Part model, mm, in its own coordinate system. Face numbers are marked on the shaded views. A direction names the side the tool comes from. Give positions to 0.01 mm unless a question says otherwise; leave off trailing zeros. Write each loop counter-clockwise with the first axis right and the second up, starting at its lowest first coordinate (ties: lowest second). Pieces come first, ordered by that corner, then holes. Notation, with made-up numbers: M -19.75,10 L 15.25,10 A18 ccw 15.25,22 Z; hole C -10.75,62.5 d11. An arc over 180 degrees is marked long. Use a Markdown table: item, result.
```python
from build123d import *

# Parameters (mm, degrees)
SKETCH1_W               = 139.999999908
SKETCH1_H               = 52.6999962
BOSS_EXTRUDE1_DEPTH     = 33.02
CUT_EXTRUDE1_DEPTH      = 154.191416123
CUT_EXTRUDE1_DEPTH_BACK = 154.191416123
CUT_EXTRUDE2_DEPTH      = 26
CUT_EXTRUDE3_START      = -26
CUT_EXTRUDE3_DEPTH      = 26
CUT_EXTRUDE4_DEPTH      = 154.191416123
CUT_EXTRUDE4_DEPTH_BACK = 154.191416123
SKETCH6_W               = 26
SKETCH6_H               = 36
CUT_EXTRUDE5_DEPTH      = 154.191416123
CUT_EXTRUDE5_DEPTH_BACK = 154.191416123
SKETCH7_R               = 1.500000048
SKETCH7_R_2             = 1.5


with BuildPart() as part:
    # Sketch1 → Boss-Extrude1 (new body)
    with BuildSketch(Plane.XY):
        with Locations((69.999999954, 26.3499981)):
            Rectangle(SKETCH1_W, SKETCH1_H)
    extrude(amount=BOSS_EXTRUDE1_DEPTH)

    # Sketch2 → Cut-Extrude1 (cut, two sides: drawn at the far end of the back side and taken through both)
    with BuildSketch(Plane.ZY.offset(-CUT_EXTRUDE1_DEPTH_BACK)):
        with BuildLine():
            Line((33.02, 44.3499981), (33.02, 8.3499981))
            ThreePointArc((33.02, 8.3499981), (15.02, 26.3499981), (33.02, 44.3499981))
        make_face()
    extrude(amount=CUT_EXTRUDE1_DEPTH + CUT_EXTRUDE1_DEPTH_BACK, mode=Mode.SUBTRACT)

    # Sketch3 → Cut-Extrude2 (cut)
    with BuildSketch(Plane.ZY):
        with BuildLine():
            Line((33.02, 46.3499981), (33.02, 6.3499981))
            ThreePointArc((33.02, 6.3499981), (13.02, 26.3499981), (33.02, 46.3499981))
        make_face()
    extrude(amount=-CUT_EXTRUDE2_DEPTH, mode=Mode.SUBTRACT)

    # Sketch5 → Cut-Extrude3 (cut)
    with BuildSketch(Plane(origin=(139.999999908, 0, 0), x_dir=(0, 0, -1), z_dir=(1, 0, 0)).offset(CUT_EXTRUDE3_START)):
        with BuildLine():
            Line((-33.02, 46.3499981), (-33.02, 6.3499981))
            ThreePointArc((-33.02, 6.3499981), (-13.02, 26.3499981), (-33.02, 46.3499981))
        make_face()
    extrude(amount=CUT_EXTRUDE3_DEPTH, mode=Mode.SUBTRACT)

    # Sketch6 → Cut-Extrude4 (cut, two sides: drawn at the far end of the back side and taken through both)
    with BuildSketch(Plane(origin=(0, 0, 0), x_dir=(-1, 0, 0), z_dir=(0, 0, -1)).offset(-CUT_EXTRUDE4_DEPTH_BACK)):
        with Locations((-69.999999954, 26.3499981)):
            Rectangle(SKETCH6_W, SKETCH6_H)
    extrude(amount=CUT_EXTRUDE4_DEPTH + CUT_EXTRUDE4_DEPTH_BACK, mode=Mode.SUBTRACT)

    # Sketch7 → Cut-Extrude5 (cut, two sides: drawn at the far end of the back side and taken through both)
    with BuildSketch(Plane.XY.offset(33.02).offset(-CUT_EXTRUDE5_DEPTH_BACK)):
        with Locations((6.35, 49.52499715)):
            Circle(SKETCH7_R)
        with Locations((6.35, 3.17499905)):
            Circle(SKETCH7_R_2)
        with Locations((133.649999908, 49.52499715)):
            Circle(SKETCH7_R_2)
        with Locations((133.649999908, 3.17499905)):
            Circle(SKETCH7_R_2)
    extrude(amount=CUT_EXTRUDE5_DEPTH + CUT_EXTRUDE5_DEPTH_BACK, mode=Mode.SUBTRACT)


solid = part.part
```
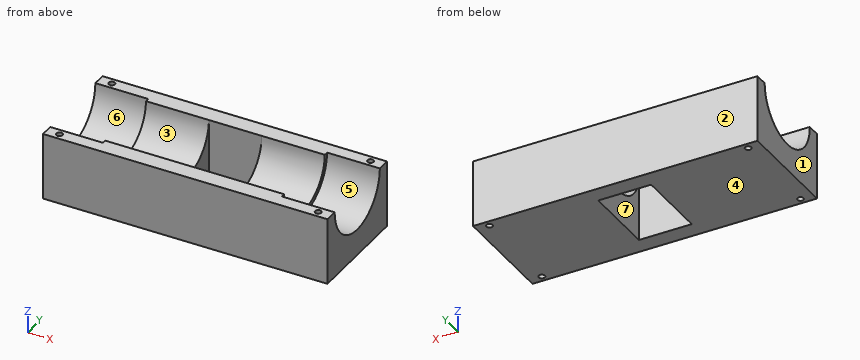
1. Tool access for the marked faces 4, 5, 6 and 7: list every direction of +Z, -Z, +X, -X, +Y, -Y with a clear straight run to the whole face (end or side of a thin tool).
Findings below:
| item | result |
|---|---|
| face 4 | -Z, +X, -X, +Y, -Y |
| face 5 | +Z, +X |
| face 6 | +Z, -X |
| face 7 | +Z, -Z |
2. Cut at C-C, the plane x = 133.65. Give the cut face in (y, z) (3 decimals), then the cut area to 3 significant figures.
Findings below:
| item | result |
|---|---|
| outline | M 0,0 L 1.675,0 L 1.675,33.02 L 0,33.02 Z; M 4.675,0 L 48.025,0 L 48.025,33.02 L 46.35,33.02 A20 cw 6.35,33.02 L 4.675,33.02 Z; M 51.025,0 L 52.7,0 L 52.7,33.02 L 51.025,33.02 Z |
| area | 914 mm2 |
3. Cut at A-A, the plane x = 65. Give the cut face in (y, z).
Findings below:
| item | result |
|---|---|
| outline | M 0,0 L 8.35,0 L 8.35,33.02 L 0,33.02 Z; M 44.35,0 L 52.7,0 L 52.7,33.02 L 44.35,33.02 Z |
4. Cut at D-D, the plane y = 31. Give the cut face in (x, z), then the cut area to 3 significant figures.
Findings below:
| item | result |
|---|---|
| outline | M 0,0 L 57,0 L 57,15.63 L 26,15.63 L 26,13.57 L 0,13.57 Z; M 83,0 L 140,0 L 140,13.57 L 114,13.57 L 114,15.63 L 83,15.63 Z |
| area | 1,670 mm2 |
5. Drop flat-ended pins along their axis: P1, Ø1.8, axis at x = 6.35, y = 3.175, coming from the -Z side; P2, Ø1.5, axis at x = 45, y = 41.5, coming from the +Z side; P3, Ø1.5, axis at x = 90.5, y = 30, coming from the +Z side. Give the stop position or say it passes through.
Findings below:
| item | result |
|---|---|
| P1 | through |
| P2 | z = 24.58 |
| P3 | z = 15.57 |
6. Drill centre lines: L1, parallel to X at y = 3, z = 18; L2, parallel to Y at x = 133.65, z = 8 (3 decimals); L3, parallel to Y at x = 69, z = 17.5. Where is each one in solid material? Low to high.
Findings below:
| item | result |
|---|---|
| L1 | 0 to 4.86, 7.84 to 132.16, 135.14 to 140 |
| L2 | 0 to 1.675, 4.675 to 48.025, 51.025 to 52.7 |
| L3 | 0 to 8.35, 44.35 to 52.7 |
7. Two-plate mould, pull along Y, no slides. Class the marked faces 1, 2 and 3: released by +Y, released by -Y, zero draft, split by the parting line, or undercut.
Findings below:
| item | result |
|---|---|
| face 1 | zero draft |
| face 2 | released by +Y |
| face 3 | undercut |
8. Cut at B-B, the plane z = 26. State how many separate pieces and enclosed holes the cut face has, then the cut area to 3 significant figures.
Findings below:
| item | result |
|---|---|
| separate pieces | 2 |
| enclosed holes | 4 |
| area | 2,410 mm2 |
